from build123d import *

# Parameters (mm, degrees)
PAD_DEPTH          = 8.5
POCKET_DEPTH       = 3
POCKET001_DEPTH    = 3
SKETCH003_W        = 17
SKETCH003_H        = 11
POCKET002_DEPTH    = 17.001
SKETCH004_W        = 1.5
SKETCH004_H        = 4
PAD001_DEPTH       = 1
POLARPATTERN_COUNT = 2
POLARPATTERN_ANGLE = 90
CHAMFER_SIZE       = 0.25


with BuildPart() as part:
    # Sketch → Pad (new body, symmetric)
    with BuildSketch(Plane.XZ):
        Polygon((-10, 10), (-10, -10), (10, -10), (10, -7), (-7, 10), align=None)
    extrude(amount=PAD_DEPTH, both=True)

    # Sketch001 (on Face1 of Pad) → Pocket (cut)
    with BuildSketch(Plane(origin=(-10, 0, 0), x_dir=(0, 0, -1), z_dir=(-1, 0, 0))):
        with BuildLine():
            ThreePointArc((-1.5, 2.9), (-4.4, 0), (-1.5, -2.9))
            Line((-1.5, -2.9), (1.5, -2.9))
            ThreePointArc((1.5, -2.9), (4.4, 0), (1.5, 2.9))
            Line((1.5, 2.9), (-1.5, 2.9))
        make_face()
    extrude(amount=-POCKET_DEPTH, mode=Mode.SUBTRACT)

    # Sketch002 (on Face5 of Pocket) → Pocket001 (cut)
    with BuildSketch(Plane(origin=(0, 0, -10), x_dir=(1, 0, 0), z_dir=(0, 0, -1))):
        with BuildLine():
            ThreePointArc((-1.5, 2.9), (-4.4, 0), (-1.5, -2.9))
            Line((-1.5, -2.9), (1.5, -2.9))
            ThreePointArc((1.5, -2.9), (4.4, 0), (1.5, 2.9))
            Line((1.5, 2.9), (-1.5, 2.9))
        make_face()
    extrude(amount=-POCKET001_DEPTH, mode=Mode.SUBTRACT)

    # Sketch003 (on Face17 of Pocket001) → Pocket002 (cut, through all)
    with BuildSketch(Plane(origin=(0, 0, -7), x_dir=(1, 0, 0), z_dir=(0, 0, -1))):
        with Locations((1.5, 0)):
            Rectangle(SKETCH003_W, SKETCH003_H)
    extrude(amount=-POCKET002_DEPTH, mode=Mode.SUBTRACT)

    # Sketch004 (on Face1 of Pocket002) → Pad001 (join)
    with BuildSketch(Plane(origin=(-10, 0, 0), x_dir=(0, 0, -1), z_dir=(-1, 0, 0))):
        with Locations((-7.75, 0)):
            Rectangle(SKETCH004_W, SKETCH004_H)
        with Locations((7.75, 0)):
            Rectangle(SKETCH004_W, SKETCH004_H)
    pad001 = extrude(amount=PAD001_DEPTH)

    # PolarPattern: Pad001 ×2 about axis
    polarpattern_axis = Axis((0, 0, 0), (0, -1, 0))
    for i in range(1, POLARPATTERN_COUNT):
        add(pad001.rotate(polarpattern_axis, i * POLARPATTERN_ANGLE / (POLARPATTERN_COUNT - 1)))

    # Chamfer
    chamfer_edges = [part.edges().sort_by_distance(p)[0] for p in [
        (-11, 0, 8.5),
        (-11, 0, 7),
        (-11, 0, -7),
        (-11, 0, -8.5),
        (-8.5, 0, -11),
        (-7, 0, -11),
        (7, 0, -11),
        (8.5, 0, -11),
    ]]
    chamfer(chamfer_edges, length=CHAMFER_SIZE)


solid = part.part
Verification items for the finished model (mm, model axes). A direction names the side the tool comes from. Coordinates: 2 decimals unless noted, no trailing zeros. Order: outer loops, then holes, each group sorted by start corner. A loop starts at its lowest first (then second) coordinate and runs counter-clockwise, first axis right, second up.
Item 1: Section check D-D, the plane y = 0. Give the number of separate pieces and of enclosed holes in the cut face, then the cut area to 4 significant figures.
Filled in:
separate pieces: 3
enclosed holes: 0
area: 63.95 mm2
Item 2: Material ranges on L1, parallel to Y at x = 0.75, z = -0.25; L2, parallel to X at y = -7, z = -9.5; L3, parallel to Z at x = -0.5, y = -3.5, recorded low to high.
Filled in:
L1: y = -8.5 to -5.5, 5.5 to 8.5
L2: x = -10 to 10
L3: z = -10 to -7
Item 3: Section check B-B, the plane x = 5.5. Enter the section's corners in (y, z).
Filled in:
outline: (-8.5, -10) - (8.5, -10) - (8.5, -2.5) - (5.5, -2.5) - (5.5, -7) - (-5.5, -7) - (-5.5, -2.5) - (-8.5, -2.5) - close
Item 4: Section check A-A, the plane z = -0.5. Enter the section's corners in (x, y), then the cut area to 3 significant figures.
Filled in:
outline: (-10, -8.5) - (3.5, -8.5) - (3.5, -5.5) - (-7, -5.5) - (-7, -2.9) - (-10, -2.9) - close; (-10, 2.9) - (-7, 2.9) - (-7, 5.5) - (3.5, 5.5) - (3.5, 8.5) - (-10, 8.5) - close
area: 96.6 mm2
Item 5: Release check for a two-part mould opening along Y. For faces 1 (the face through (2, 7, 1)), 2 (the face through (-2, 8.5, -2)), 3 (the face through (0, -2.9, -9)) record: +Y half, -Y half, draft (parallel to the pull), parting line (faces both ways), or undercut.
Filled in:
face 1: draft
face 2: +Y half
face 3: undercut
Item 6: Section check C-C, the plane y = 7.25. Enter the section's corners in (x, z).
Filled in:
outline: (-10, -10) - (10, -10) - (10, -7) - (-7, 10) - (-10, 10) - close
Item 7: Access from +Z, -Z, +X, -X, +Y, -Y to the whole of each face (thin tool, end or side, straight path). Record for faces 4 (the face through (-10.5, 2, 7.8)), 5 (the face through (7.7, 2, -10.5)), 6 (the face through (-10.5, -2, -7.7)), 7 (the face through (-1, 5.5, -1)).
Filled in:
face 4: +Z, -Z, -X, +Y
face 5: -Z, +X, -X, +Y
face 6: +Z, -Z, -X, -Y
face 7: +Z, +X
Item 8: Depth check by flat-ended pin: pin 1 (0.8 mm diameter, centred on y = -1, z = -10.5, fed in from -X); pin 2 (1.5 mm diameter, centred on x = -2, z = 6.5, fed in from -Y); pin 3 (0.8 mm diameter, centred on x = -8, z = -10.5, fed in from -Y); pin 4 (1 mm diameter, centred on x = 2.5, y = 6, fed in from -Z). Enter the tip coordinate at first touch or a pass-through.
Filled in:
pin 1: stops at x = -8.5
pin 2: passes through
pin 3: stops at y = -2
pin 4: stops at z = -10
